Model file for the job. Use its own axes, mm. A direction names the side the tool comes from. Coordinates: 2 decimals unless noted, no trailing zeros. Order: outer loops, then holes, each group sorted by start corner. A loop starts at its lowest first (then second) coordinate and runs counter-clockwise, first axis right, second up. Notation, with made-up numbers: (88, 44.5) -> (141, 44.5) arc R29 ccw to (141, 74.5) -> close; hole circle Ø11 at (37, -34). An arc over 180 degrees is marked (long way). Write item = value, one per line. Start each with the question number.
Q1. Flat gauge pins, fed straight in: pin 1 (3.5 mm diameter, centred on x = -50.05, y = -15, fed in from -Z); pin 2 (1 mm diameter, centred on x = -54, y = -25, fed in from +Z); pin 3 (2 mm diameter, centred on x = -48.5, y = -22, fed in from +Z); pin 4 (1 mm diameter, centred on x = -47, z = 25.5, fed in from +Y). Where does each tip first touch, or does it go through?
Q2. Cut at A-A, the plane z = 21.75. List the corners of the cut face in (x, y), plus the area to 3 significant figures.
Q3. Cut at D-D, the plane z = 25.25. List the corners of the cut face in (x, y).
Q4. Mould opens along Y. For faces 4 (the face through (-50, -15, 25.896)), 5 (the face through (-47.513, -15, 22)), 6 (the face through (-50, -30, 24)), 7 (the face through (-52.048, -15.088, 23.361)) say: +Y half, -Y half, draft (parallel to the pull), parting line (faces both ways), or undercut.
Q5. Wall check: line 1 (X direction, y = -15, z = 24); line 2 (Z direction, x = -51.5, y = -19); line 3 (Y direction, x = -49, z = 25.75). Give the ranges that are in metal, low to high. Write a range as from..to.
Q6. Cut at B-B, the plane y = -15. List the corners of the cut face in (x, z).
Q7. Cut at C-C, the plane x = -46.25. List the corners of the cut face in (y, z).
Q8. 3-axis set-ups, long thin cutter, end or side, ignore diameter. For faces 1 (the face through (-53.013, -15, 22)), 2 (the face through (-46, -15, 22.896)), 3 (the face through (-49, -15, 27.054)): which of +Z, -Z, +X, -X, +Y, -Y reach the whole face in a straight line?
from build123d import *

# Parameters (mm, degrees)
F1_DEPTH = 30
F2_R     = 2
F3_DEPTH = 5


with BuildPart() as f1:
    # F0 (on Front) → F1 (new body)
    with BuildSketch(Plane.XZ):
        with BuildLine():
            Line((-50.474065, 27.053742), (-53.244065, 27.053742))
            Line((-53.244065, 27.053742), (-55.761366, 24.536442))
            Line((-55.761366, 24.536442), (-55.761366, 22.896442))
            Line((-55.761366, 22.896442), (-53.012501, 22.896442))
            Line((-53.012501, 22.896442), (-53.012501, 21.223109))
            ThreePointArc((-53.012501, 21.223109), (-52.916823, 20.99212), (-52.685834, 20.896442))
            Line((-52.685834, 20.896442), (-47.839168, 20.896442))
            ThreePointArc((-47.839168, 20.896442), (-47.60818, 20.99212), (-47.512501, 21.223109))
            Line((-47.512501, 21.223109), (-47.512501, 22.896442))
            Line((-47.512501, 22.896442), (-44.762501, 22.896442))
            Line((-44.762501, 22.896442), (-44.762501, 24.536442))
            Line((-44.762501, 24.536442), (-47.279801, 27.053742))
            Line((-47.279801, 27.053742), (-50.049801, 27.053742))
            Line((-50.049801, 27.053742), (-50.261933, 27.265874))
            Line((-50.261933, 27.265874), (-50.474065, 27.053742))
        make_face()
    extrude(amount=F1_DEPTH)

    # F2 (on face) → F3 (cut)
    with BuildSketch(Plane(origin=(0, 0, 20.896442), x_dir=(1, 0, 0), z_dir=(0, 0, -1))):
        with Locations((-50.049801, 15)):
            Circle(F2_R)
    extrude(amount=-F3_DEPTH, mode=Mode.SUBTRACT)


solid = f1.part
Here are the results:
q1.pin_1 = 25.9
q1.pin_2 = 26.8
q1.pin_3 = 27.05
q1.pin_4 = 0
q2.outline = (-53.01, -30) -> (-47.51, -30) -> (-47.51, 0) -> (-53.01, 0) -> close; hole circle Ø4 at (-50.05, -15)
q2.area = 152 mm²
q3.outline = (-55.05, -30) -> (-45.48, -30) -> (-45.48, 0) -> (-55.05, 0) -> close; hole circle Ø4 at (-50.05, -15)
q4.face_4 = undercut
q4.face_5 = draft
q4.face_6 = -Y half
q4.face_7 = undercut
q5.line_1 = -55.76..-52.05, -48.05..-44.76
q5.line_2 = 20.9..27.05
q5.line_3 = -30..-16.7, -13.3..0
q6.outline = (-55.76, 22.9) -> (-53.01, 22.9) -> (-53.01, 21.22) arc R0.33 ccw to (-52.69, 20.9) -> (-52.05, 20.9) -> (-52.05, 25.9) -> (-48.05, 25.9) -> (-48.05, 20.9) -> (-47.84, 20.9) arc R0.33 ccw to (-47.51, 21.22) -> (-47.51, 22.9) -> (-44.76, 22.9) -> (-44.76, 24.54) -> (-47.28, 27.05) -> (-50.05, 27.05) -> (-50.26, 27.27) -> (-50.47, 27.05) -> (-53.24, 27.05) -> (-55.76, 24.54) -> close
q7.outline = (-30, 22.9) -> (0, 22.9) -> (0, 26.02) -> (-30, 26.02) -> close
q8.face_1 = -Z, -X, +Y, -Y
q8.face_2 = -Z, +X, +Y, -Y
q8.face_3 = +Z, +X, +Y, -Y
